Autodesk Inventor part; units mm, degrees
ref_plane "YZ Plane" through (0, 0, 0) normal (1, 0, 0) x (0, 1, 0)
ref_plane "XZ Plane" through (0, 0, 0) normal (0, 1, 0) x (-1, 0, 0)
ref_plane "XY Plane" through (0, 0, 0) normal (0, 0, 1) x (1, 0, 0)
sketch "Esboço1" plane through (0, 0, 0) normal (0, 1, 0) x (-1, 0, 0)
  line L0 (-5, 5) -> (5, 5)
  line L1 (5, 5) -> (5, -5)
  line L2 (5, -5) -> (-5, -5)
  line L3 (-5, -5) -> (-5, 5)
  line L4 (-5, 5) -> (5, -5) construction
  line L5 (5, 5) -> (-5, -5) construction
  point P0 (0, 0)
  dimension "d0" = 10
  dimension "d1" = 10
extrude "Extrusão1" add sketch "Esboço1" along normal blind 6
sketch "Esboço2" plane through (5, 0, 5) normal (1, 0, 0) x (0, 0, -1)
  line L0 (2, 0) -> (2, 1.5)
  line L1 (0, 0) -> (0, 6)
  line L2 (2, 1.5) -> (8, 1.5)
  line L3 (8, 1.5) -> (8, 0)
  line L4 (10, 0) -> (10, 6)
  line L5 (0, 0) -> (10, 0)
  point P0 (5, 0)
  dimension "d4" = 2
  dimension "d5" = 1.5
  dimension "d6" = 2
  dimension "d7" = 1.5
extrude "Extrusão2" cut sketch "Esboço2" against normal through all
sketch "Esboço3" plane through (-5, 0, 5) normal (0, 0, 1) x (1, 0, 0)
  line L0 (10, 0) -> (0, 0)
  arc A0 (8, 0) -> (2.5, 3.9823) centre (2.7087, -1.5186) ccw
  line L1 (0, 0) -> (0, 6)
  line L2 (2.5, 3.9823) -> (2.5, 0)
  point P0 (5, 0)
  dimension "d10" = 2
  dimension "d11" = 2.5
  dimension "d12" = 5.5049
  dimension "d13" = 2.7087
extrude "Extrusão3" cut sketch "Esboço3" against normal through all
sketch "Esboço4" plane through (-5, 6, 5) normal (0, 0, 1) x (1, 0, 0)
  point P0 (5, -6)
fillet "Arredondamento1" radius 1 1 edges at (-2.5, 3.9823, 0)
fillet "Arredondamento2" radius 1 2 edges at (-2.5, 0, 4) (-2.5, 0, -4)
fillet "Arredondamento3" radius 2 3 edges at (-5, 6, 0) (-5, 0, -4) (-5, 0, 4)
sketch "Esboço5" plane through (5, 0, 5) normal (0, 0, 1) x (1, 0, 0)
  circle A0 centre (-8.8, 4.5) radius 0.75
  line L0 (0, 0) -> (0, 6)
  point P0 (-5, 0)
  dimension "d19" = 1.5
  dimension "d20" = 8.8
  dimension "d21" = 4.5
extrude "Extrusão4" cut sketch "Esboço5" against normal through all
sketch "Esboço6" plane through (0, 6, 0) normal (0, 1, 0) x (1, 0, 0)
  line L0 (-5, 5) -> (-5, -5)
  line L1 (-5, 4) -> (3.5, 4)
  line L2 (5, -5) -> (5, 5)
  line L3 (3.5, -4) -> (-5, -4)
  line L4 (-5, -4) -> (-5, 4)
  line L5 (5, 5) -> (-3, 5)
  line L6 (-3, -5) -> (5, -5)
  line L7 (3.5, 4) -> (3.5, -4)
  point P0 (0, 0)
  dimension "d24" = 1
  dimension "d25" = 1
  dimension "d26" = 1.5
extrude "Extrusão5" cut sketch "Esboço6" against normal through all
sketch "Esboço7" plane through (5, 0, -5) normal (1, 0, 0) x (0, 0, -1)
  line L0 (-1, 6) -> (-9, 6)
  arc A0 (-7.5, 6) -> (-2.5, 6) centre (-5, 7.9975) ccw
  line L1 (-10, 0) -> (-10, 6)
  line L2 (0, 0) -> (0, 6)
  point P0 (-5, 0)
  dimension "d29" = 3.2
  dimension "d30" = 2.5
  dimension "d31" = 2.5
extrude "Extrusão6" cut sketch "Esboço7" against normal blind 6
properties material "Liga de Nickel-Copper 400"
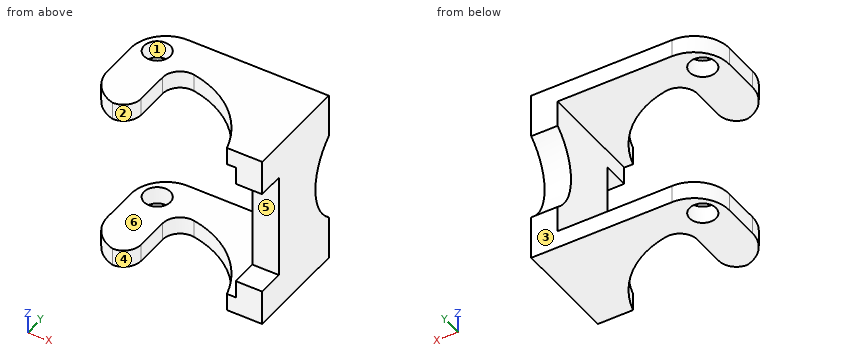
Source: CAD feature listing. Evaluate the final solid. Frame: model axes, mm. Face numbers are marked on the shaded views. A direction names the side the tool comes from. Give positions to 0.01 mm unless a question says otherwise; leave off trailing zeros. Write each loop counter-clockwise with the first axis right and the second up, starting at its lowest first coordinate (ties: lowest second). Pieces come first, ordered by that corner, then holes. Notation, with made-up numbers: (-12.5, 60) - (11.5, 60) arc R24 cw to (11.5, 76) - close; hole circle Ø8 at (74, -30). An arc over 180 degrees is marked (long way). Write item = value, one per line. Start each with the question number.
Q1. Cut plane C-C, the plane x = -3.8. Return loops of the section in (y, z).
Q2. Cut plane D-D, the plane x = 4. Return loops of the section in (y, z).
Q3. Reachability of the marked faces 4, 5 and 6 from +Z, -Z, +X, -X, +Y, -Y: full face, straight path, thin tool, end or side. Return the list, or none.
Q4. Cut plane B-B, the plane y = 4.5. Return loops of the section in (x, z), then the cut area to 3 significant figures.
Q5. Cut plane A-A, the plane x = -2. Return loops of the section in (y, z).
Q6. Pin query (flat end, axial travel): pin 1 Ø2 at (x, y) = (0.5, 0.5) entering from -Z; pin 2 Ø3 at (y, z) = (2.5, -0.5) entering from -X. Return the tip coordinate at first contact, or that it passes through.
Q7. Material intervals for probe 1 along Z at (x, y) = (-3.5, 3.65); probe 2 along X at (y, z) = (2.1, 3.75); probe 3 along Y at (x, z) = (-3.8, -4.6), sorted ascending.
Q8. Draft query along Y for the marked faces 1, 2 and 3. Return one class per face: +Y half, -Y half, draft (parallel to the pull), parting line (faces both ways), or undercut.
Computed values:
q1.outline = (0.1, -5) - (3.75, -5) - (3.75, -4) - (0.1, -4) - close; (0.1, 4) - (3.75, 4) - (3.75, 5) - (0.1, 5) - close; (5.25, -5) - (5.83, -5) - (5.83, -4) - (5.25, -4) - close; (5.25, 4) - (5.83, 4) - (5.83, 5) - (5.25, 5) - close
q2.outline = (0, -5) - (6, -5) - (6, -2.5) arc R3.2 cw to (6, 2.5) - (6, 5) - (0, 5) - (0, 3) - (1.5, 3) - (1.5, -3) - (0, -3) - close
q3.face_4 = +Z, -Z, -Y
q3.face_5 = +X, -X, -Y
q3.face_6 = -X, +Y, -Y
q4.outline = (-4.94, -5) - (-4.55, -5) - (-4.55, -4) - (-4.94, -4) - close; (-4.94, 4) - (-4.55, 4) - (-4.55, 5) - (-4.94, 5) - close; (-3.05, -5) - (5, -5) - (5, 5) - (-3.05, 5) - (-3.05, 4) - (3.5, 4) - (3.5, -4) - (-3.05, -4) - close
q4.area = 28.9 mm²
q5.outline = (3.78, -5) - (6, -5) - (6, -4) - (3.78, -4) - close; (3.78, 4) - (6, 4) - (6, 5) - (3.78, 5) - close
q6.pin_1 = through
q6.pin_2 = 3.5
q7.probe_1 = -5 to -4, 4 to 5
q7.probe_2 = 3.5 to 5
q7.probe_3 = 0.1 to 3.75, 5.25 to 5.83
q8.face_1 = undercut
q8.face_2 = -Y half
q8.face_3 = +Y half
